For this review, take the finished solid that the model builds, in its own axes (mm). A direction names the side the tool comes from. Coordinates: 2 decimals unless noted, no trailing zeros. Order: outer loops, then holes, each group sorted by start corner. A loop starts at its lowest first (then second) coordinate and runs counter-clockwise, first axis right, second up. Notation, with made-up numbers: (6, 36) -> (49, 36) arc R18 ccw to (49, 67) -> close; hole circle Ø2 at (54, 6.25). An arc over 180 degrees is marked (long way). Answer as a JSON object with one key per item and string values. Group by question number.
1) Machinability: for faces 5 (the flat face through (23, 167.274, 12)), 6 (the flat face through (44, 97.274, 14)), which of the approach directions +Z, -Z, +X, -X, +Y, -Y give a long, thin tool a straight path to every point of the face, cutting with its end or side? Answer none if there is none.
2) Wall thickness on L1, parallel to Y at x = -3, z = 22.25; L2, parallel to Y at x = 31, z = 6.25; L3, parallel to Y at x = 16.5, z = 11.75: over which ranges is each line inside the solid? List them lowest first.
3) For pin 1 (8 mm diameter, centred on x = 0.5, y = 17.5, fed in from -Z); pin 2 (1.6 mm diameter, centred on x = -14.5, z = 20, fed in from +Y); pin 3 (4 mm diameter, centred on y = 119, z = 18, fed in from -X); pin 4 (6 mm diameter, centred on x = 45, z = 15, fed in from +Y), all flat-tipped, find the tip position at first contact; note any pin that passes through.
4) Add section B-B, the plane z = 13.75. Count the separate pieces of the cut face and the enclosed holes in it, then the cut area to 3 significant figures.
5) Draft analysis for pull direction X (two halves, no side actions). For faces 1 (the flat face through (21, 83, 0)), 2 (the flat face through (57.819, 81, 10)), 3 (the flat face through (29.819, 94, 14)), 4 (the flat face through (-13.181, 124, 12)), state which applies: +X half, -X half, draft (parallel to the pull), parting line (faces both ways), or undercut.
6) Add section D-D, the plane y = 36. Write out the cut boundary in (x, z), then the cut area to 3 significant figures.
7) Add section A-A, the plane y = 147.5. Write out the cut boundary in (x, z), then the cut area to 3 significant figures.
8) Add section C-C, the plane x = -8.5. Write out the cut boundary in (y, z), then the cut area to 3 significant figures.
from build123d import *

# Parameters (mm, degrees)
F3_W      = 2
F3_H      = 110
F4_DEPTH  = 3
F5_W      = 2
F5_H      = 33
F5_H_2    = 40
F5_H_3    = 27
F5_H_4    = 19
F5_H_5    = 35
F5_W_2    = 7
F5_H_6    = 2
F6_DEPTH  = 22
F7_W      = 8.2
F7_H      = 20
F7_W_2    = 30.8
F8_DEPTH  = 2
F9_W      = 12
F9_H      = 20
F9_W_2    = 20
F9_H_2    = 12
F9_W_3    = 8
F9_W_4    = 16.4
F9_W_5    = 16
F10_DEPTH = 2
F11_W     = 22
F11_H     = 14
F12_DEPTH = 2
F13_W     = 8.2
F13_H     = 20
F14_DEPTH = 2
F15_W     = 8.2
F15_H     = 20
F16_DEPTH = 2
F17_W     = 8.2
F17_H     = 20
F18_DEPTH = 2
F19_W     = 8.2
F19_H     = 20
F20_DEPTH = 2
F21_W     = 16.4
F21_H     = 20
F21_H_2   = 12
F22_DEPTH = 2
F23_SIZE  = 2


with BuildPart() as f4:
    # F3 (on Top) → F4 (new body)
    with BuildSketch(Plane.XY):
        Polygon((57.8188975325, 167.2736013268), (-13.1811024675, 167.2736013268), (-13.1811024675, 107.2736013268), (-13.1811024675, -2.7263986732), (57.8188975325, -2.7263986732), align=None)
        with Locations((-14.1811024675, 52.2736013268)):
            Rectangle(F3_W, F3_H)
    extrude(amount=F4_DEPTH)

    # F5 (on face) → F6 (join)
    with BuildSketch(Plane.XY.offset(3)):
        with Locations((56.8188975325, 15.7736013268)):
            Rectangle(F5_W, F5_H)
        with Locations((56.8188975325, 54.2736013268)):
            Rectangle(F5_W, F5_H_2)
        Polygon((-13.1811024675, 167.2736013268), (-13.1811024675, 107.2736013268), (-11.1811024675, 107.2736013268), (-11.1811024675, 165.2736013268), (-11.1811024675, 167.2736013268), align=None)
        Polygon((-11.1811024675, 167.2736013268), (-11.1811024675, 165.2736013268), (55.8188975325, 165.2736013268), (57.8188975325, 165.2736013268), (57.8188975325, 167.2736013268), align=None)
        Polygon((-15.1811024675, -0.7263986732), (-15.1811024675, -2.7263986732), (57.8188975325, -2.7263986732), (57.8188975325, -0.7263986732), (55.8188975325, -0.7263986732), (27.8188975325, -0.7263986732), (25.8188975325, -0.7263986732), (-13.1811024675, -0.7263986732), align=None)
        Polygon((-11.1811024675, 107.2736013268), (-13.1811024675, 107.2736013268), (-13.1811024675, 105.2736013268), (20.8188975325, 105.2736013268), (22.8188975325, 105.2736013268), (22.8188975325, 107.2736013268), align=None)
        Polygon((55.8188975325, 76.2736013268), (57.8188975325, 76.2736013268), (57.8188975325, 165.2736013268), (55.8188975325, 165.2736013268), (55.8188975325, 97.2736013268), (55.8188975325, 95.2736013268), align=None)
        Polygon((-15.1811024675, 107.2736013268), (-15.1811024675, -0.7263986732), (-13.1811024675, -0.7263986732), (-13.1811024675, 32.2736013268), (-13.1811024675, 34.2736013268), (-13.1811024675, 76.2736013268), (-13.1811024675, 78.2736013268), (-13.1811024675, 105.2736013268), (-13.1811024675, 107.2736013268), align=None)
        Polygon((55.8188975325, 74.2736013268), (57.8188975325, 74.2736013268), (57.8188975325, 76.2736013268), (55.8188975325, 76.2736013268), (31.8188975325, 76.2736013268), (29.8188975325, 76.2736013268), (29.8188975325, 74.2736013268), (31.8188975325, 74.2736013268), align=None)
        Polygon((55.8188975325, 32.2736013268), (57.8188975325, 32.2736013268), (57.8188975325, 34.2736013268), (55.8188975325, 34.2736013268), (31.8188975325, 34.2736013268), (29.8188975325, 34.2736013268), (22.8188975325, 34.2736013268), (20.8188975325, 34.2736013268), (-13.1811024675, 34.2736013268), (-13.1811024675, 32.2736013268), (25.8188975325, 32.2736013268), (27.8188975325, 32.2736013268), align=None)
        with Locations((21.8188975325, 91.7736013268)):
            Rectangle(F5_W, F5_H_3)
        Polygon((20.8188975325, 76.2736013268), (20.8188975325, 34.2736013268), (22.8188975325, 34.2736013268), (22.8188975325, 52.2736013268), (22.8188975325, 54.2736013268), (22.8188975325, 76.2736013268), align=None)
        Polygon((-13.1811024675, 78.2736013268), (-13.1811024675, 76.2736013268), (20.8188975325, 76.2736013268), (22.8188975325, 76.2736013268), (22.8188975325, 78.2736013268), (20.8188975325, 78.2736013268), align=None)
        with Locations((30.8188975325, 85.7736013268)):
            Rectangle(F5_W, F5_H_4)
        Polygon((55.8188975325, 95.2736013268), (55.8188975325, 97.2736013268), (31.8188975325, 97.2736013268), (29.8188975325, 97.2736013268), (29.8188975325, 95.2736013268), (31.8188975325, 95.2736013268), align=None)
        with Locations((30.8188975325, 114.7736013268)):
            Rectangle(F5_W, F5_H_5)
        Polygon((29.8188975325, 34.2736013268), (31.8188975325, 34.2736013268), (31.8188975325, 74.2736013268), (29.8188975325, 74.2736013268), (29.8188975325, 54.2736013268), (29.8188975325, 52.2736013268), align=None)
        with Locations((26.3188975325, 53.2736013268)):
            Rectangle(F5_W_2, F5_H_6)
        with Locations((26.8188975325, 15.7736013268)):
            Rectangle(F5_W, F5_H)
    extrude(amount=F6_DEPTH)

    # F7 (on face) → F8 (cut)
    with BuildSketch(Plane(origin=(-13.1811024675, 0, 0), x_dir=(0, -1, 0), z_dir=(-1, 0, 0))):
        with Locations((-116.3736013268, 13)):
            Rectangle(F7_W, F7_H)
        with Locations((-143.8736013268, 13)):
            Rectangle(F7_W_2, F7_H)
    extrude(amount=-F8_DEPTH, mode=Mode.SUBTRACT)

    # F9 (on face) → F10 (cut)
    with BuildSketch(Plane(origin=(55.8188975325, 0, 0), x_dir=(0, -1, 0), z_dir=(-1, 0, 0))):
        with Locations((-113.2736013268, 13)):
            Rectangle(F9_W, F9_H)
        with Locations((-133.2736013268, 17)):
            Rectangle(F9_W_2, F9_H_2)
        with Locations((-84.2736013268, 17)):
            Rectangle(F9_W_3, F9_H_2)
        with Locations((-58.0736013268, 13)):
            Rectangle(F9_W_4, F9_H)
        with Locations((-15.2736013268, 17)):
            Rectangle(F9_W_5, F9_H_2)
    extrude(amount=-F10_DEPTH, mode=Mode.SUBTRACT)

    # F11 (on face) → F12 (cut)
    with BuildSketch(Plane.XZ.offset(-165.2736013268)):
        with Locations((42.8188975325, 16)):
            Rectangle(F11_W, F11_H)
        with Locations((7.8188975325, 16)):
            Rectangle(F11_W, F11_H)
    extrude(amount=-F12_DEPTH, mode=Mode.SUBTRACT)

    # F13 (on face) → F14 (cut)
    with BuildSketch(Plane(origin=(20.8188975325, 0, 0), x_dir=(0, -1, 0), z_dir=(-1, 0, 0))):
        with Locations((-85.3736013268, 13)):
            Rectangle(F13_W, F13_H)
        with Locations((-64.1736013268, 13)):
            Rectangle(F13_W, F13_H)
        with Locations((-44.3736013268, 13)):
            Rectangle(F13_W, F13_H)
    extrude(amount=-F14_DEPTH, mode=Mode.SUBTRACT)

    # F15 (on face) → F16 (cut)
    with BuildSketch(Plane.YZ.offset(31.8188975325)):
        with Locations((82.3736013268, 13)):
            Rectangle(F15_W, F15_H)
        with Locations((68.1736013268, 13)):
            Rectangle(F15_W, F15_H)
    extrude(amount=-F16_DEPTH, mode=Mode.SUBTRACT)

    # F17 (on face) → F18 (cut)
    with BuildSketch(Plane.XZ.offset(-32.2736013268)):
        with Locations((43.7188975325, 13)):
            Rectangle(F17_W, F17_H)
    extrude(amount=-F18_DEPTH, mode=Mode.SUBTRACT)

    # F19 (on face) → F20 (cut)
    with BuildSketch(Plane(origin=(25.8188975325, 0, 0), x_dir=(0, -1, 0), z_dir=(-1, 0, 0))):
        with Locations((-9.3736013268, 13)):
            Rectangle(F19_W, F19_H)
    extrude(amount=-F20_DEPTH, mode=Mode.SUBTRACT)

    # F21 (on face) → F22 (cut)
    with BuildSketch(Plane.YZ.offset(-13.1811024675)):
        with Locations((13.4736013268, 13)):
            Rectangle(F21_W, F21_H)
        with Locations((50.4736013268, 17)):
            Rectangle(F21_W, F21_H_2)
        with Locations((89.4736013268, 17)):
            Rectangle(F21_W, F21_H_2)
    extrude(amount=-F22_DEPTH, mode=Mode.SUBTRACT)

    # F23
    f23_edges = [f4.edges().sort_by_distance(p)[0] for p in [
        (-12.181102, 159.273601, 23),
        (-12.181102, 128.473601, 23),
        (-12.181102, 112.273601, 23),
        (-14.181102, 81.273601, 23),
        (18.818898, 166.273601, 23),
        (-14.181102, 21.673601, 23),
        (-14.181102, 58.673601, 23),
        (-14.181102, 97.673601, 23),
        (-12.181102, 120.473601, 23),
        (-14.181102, 5.273601, 23),
        (56.818898, 7.273601, 23),
        (26.818898, 5.273601, 23),
        (56.818898, 49.873601, 23),
        (56.818898, 80.273601, 23),
        (56.818898, 23.273601, 23),
        (56.818898, 66.273601, 23),
        (56.818898, 88.273601, 23),
        (39.618898, 33.273601, 23),
        (30.818898, 72.273601, 23),
        (21.818898, 68.273601, 23),
        (26.818898, 13.473601, 23),
        (31.818898, 166.273601, 23),
        (56.818898, 123.273601, 23),
        (56.818898, 107.273601, 23),
        (56.818898, 119.273601, 23),
        (56.818898, 143.273601, 23),
        (53.818898, 166.273601, 23),
        (-3.181102, 166.273601, 23),
        (30.818898, 78.273601, 23),
        (30.818898, 86.473601, 23),
        (30.818898, 64.073601, 23),
        (21.818898, 89.473601, 23),
        (21.818898, 81.273601, 23),
        (21.818898, 40.273601, 23),
        (21.818898, 48.473601, 23),
        (21.818898, 60.073601, 23),
    ]]
    chamfer(f23_edges, length=F23_SIZE)


solid = f4.part
Output values:
{
 "1": {"face 5": "+Z, -Z, +X, -X, +Y", "face 6": "+Z"},
 "2": {"L1": "y = -2.73 to -0.73, 32.27 to 34.27, 76.27 to 78.27, 105.27 to 107.27, 165.27 to 167.27", "L2": "y = -2.73 to -0.73, 32.27 to 64.07, 72.27 to 78.27, 86.47 to 132.27, 165.27 to 167.27", "L3": "y = -2.73 to -0.73, 32.27 to 34.27, 76.27 to 78.27, 105.27 to 107.27"},
 "3": {"pin 1": "stops at z = 0", "pin 2": "stops at y = 107.27", "pin 3": "stops at x = -13.18", "pin 4": "stops at y = 97.27"},
 "4": {"separate pieces": "12", "enclosed holes": "0", "area": "1,220 mm²"},
 "5": {"face 1": "draft", "face 2": "+X half", "face 3": "undercut", "face 4": "-X half"},
 "6": {"outline": "(-15.18, 0) -> (57.82, 0) -> (57.82, 25) -> (55.82, 25) -> (55.82, 3) -> (31.82, 3) -> (31.82, 25) -> (29.82, 25) -> (29.82, 3) -> (22.82, 3) -> (22.82, 25) -> (20.82, 25) -> (20.82, 3) -> (-13.18, 3) -> (-13.18, 25) -> (-15.18, 25) -> close", "area": "395 mm²"},
 "7": {"outline": "(-13.18, 0) -> (57.82, 0) -> (57.82, 25) -> (55.82, 25) -> (55.82, 3) -> (-13.18, 3) -> close; (-13.18, 23) -> (-11.18, 23) -> (-11.18, 25) -> (-13.18, 25) -> close", "area": "261 mm²"},
 "8": {"outline": "(-2.73, 0) -> (167.27, 0) -> (167.27, 25) -> (165.27, 25) -> (165.27, 3) -> (107.27, 3) -> (107.27, 25) -> (105.27, 25) -> (105.27, 3) -> (78.27, 3) -> (78.27, 25) -> (76.27, 25) -> (76.27, 3) -> (34.27, 3) -> (34.27, 25) -> (32.27, 25) -> (32.27, 3) -> (-0.73, 3) -> (-0.73, 25) -> (-2.73, 25) -> close", "area": "730 mm²"}
}
